Drawing for the job (mm, zero at the part's lowest x, y, z). A direction names the side the tool comes from. Coordinates: 2 decimals unless noted, no trailing zeros. Order: outer loops, then holes, each group sorted by start corner. A loop starts at its lowest first (then second) coordinate and runs counter-clockwise, first axis right, second up.
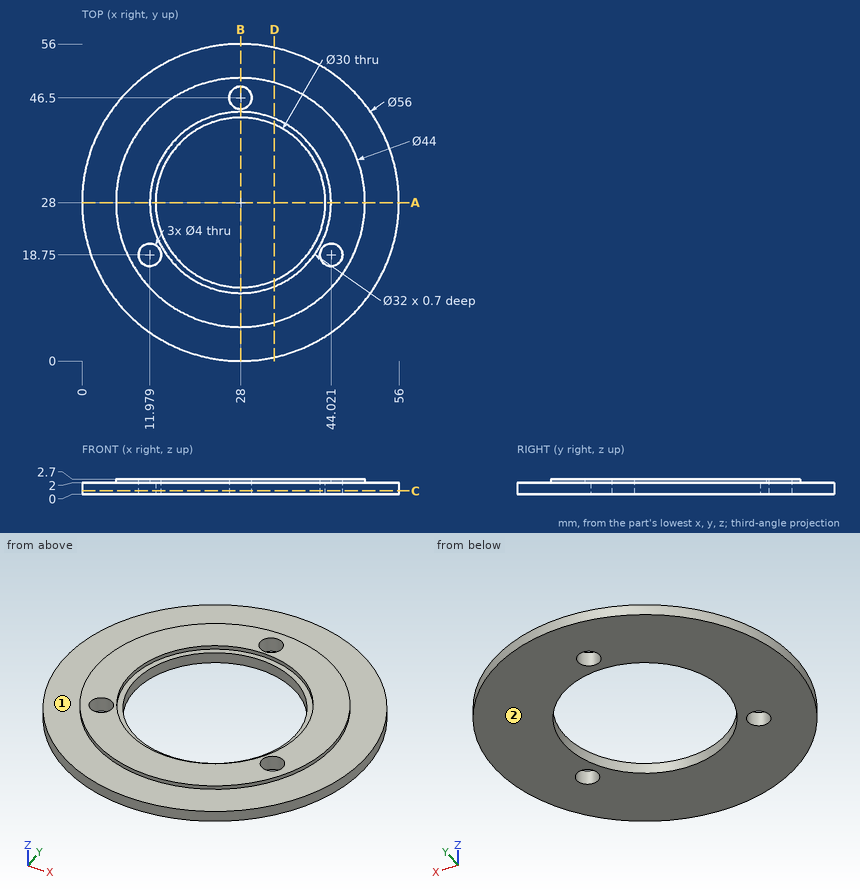
(1) Probe line 1 (Y direction, x = 28, z = 2.4); line 2 (Y direction, x = 28, z = 1.2); line 3 (X direction, y = 18.75, z = 1.45). List the from-to ranges inside material, lowest first.
(2) Drop a flat-ended pin along its axis: pin 1 (1.5 mm diameter, centred on x = 26, z = 1.5, fed in from -Y). Give the stop position or say it passes through.
(3) Tool access for the marked faces 1 and 2: list every direction of +Z, -Z, +X, -X, +Y, -Y with a clear straight run to the whole face (end or side of a thin tool).
(4) Slice it at B-B, the plane x = 28. Give the cut face in (y, z).
(5) Slice it at A-A, the plane y = 28. Give the cut face in (x, z).
(6) Slice it at D-D, the plane x = 34. Give the cut face in (y, z).
(7) Slice it at C-C, the plane z = 0.6. Give the cut face in (x, y).
Here are the results:
1. line 1: y = 6 to 12, 44 to 44.5, 48.5 to 50
1. line 2: y = 0 to 13, 43 to 44.5, 48.5 to 56
1. line 3: x = 1.57 to 9.98, 13.98 to 16.19, 39.81 to 42.02, 46.02 to 54.43
2. pin 1: stops at y = 0.03
3. face 1: +Z
3. face 2: -Z, +X, -X, +Y, -Y
4. outline: (0, 0) - (13, 0) - (13, 2) - (12, 2) - (12, 2.7) - (6, 2.7) - (6, 2) - (0, 2) - close; (43, 0) - (44.5, 0) - (44.5, 2.7) - (44, 2.7) - (44, 2) - (43, 2) - close; (48.5, 0) - (56, 0) - (56, 2) - (50, 2) - (50, 2.7) - (48.5, 2.7) - close
5. outline: (0, 0) - (13, 0) - (13, 2) - (12, 2) - (12, 2.7) - (6, 2.7) - (6, 2) - (0, 2) - close; (43, 0) - (56, 0) - (56, 2) - (50, 2) - (50, 2.7) - (44, 2.7) - (44, 2) - (43, 2) - close
6. outline: (0.65, 0) - (14.25, 0) - (14.25, 2) - (13.17, 2) - (13.17, 2.7) - (6.83, 2.7) - (6.83, 2) - (0.65, 2) - close; (41.75, 0) - (55.35, 0) - (55.35, 2) - (49.17, 2) - (49.17, 2.7) - (42.83, 2.7) - (42.83, 2) - (41.75, 2) - close
7. outline: circle Ø56 at (28, 28); hole circle Ø4 at (11.98, 18.75); hole circle Ø30 at (28, 28); hole circle Ø4 at (28, 46.5); hole circle Ø4 at (44.02, 18.75)
